CAD build for the part. Positions are in the model's coordinates, mm. Face numbers are marked on the shaded views. Give positions to 0.01 mm unless a question says otherwise; leave off trailing zeros. Loops run counter-clockwise (first coordinate to the right, second up) from the corner with the lowest first, then second, coordinate; pieces in that order, holes last.
```python
from build123d import *

# Parameters (mm, degrees)
SKETCH1_R           = 1
BOSS_EXTRUDE1_DEPTH = 2
SKETCH4_W           = 2
SKETCH4_H           = 2
BOSS_EXTRUDE2_DEPTH = 12


with BuildPart() as part:
    # Sketch1 → Boss-Extrude1 (new body)
    with BuildSketch(Plane(origin=(0, 0, 0), x_dir=(1, 0, 0), z_dir=(0, 1, 0))):
        with BuildLine():
            Line((-10, 2.5), (0, 2.5))
            Line((0, 2.5), (0, -2.5))
            Line((0, -2.5), (-10, -2.5))
            ThreePointArc((-10, -2.5), (-12.5, 0), (-10, 2.5))
        make_face()
        with Locations(Location((-10, 0, 0), (0, 0, 270))):
            Circle(SKETCH1_R, mode=Mode.SUBTRACT)
    extrude(amount=BOSS_EXTRUDE1_DEPTH)

    # Sketch4 → Boss-Extrude2 (add)
    with BuildSketch(Plane(origin=(0, 0, 0), x_dir=(0, 0, -1), z_dir=(1, 0, 0))):
        with Locations((0, 1)):
            Rectangle(SKETCH4_W, SKETCH4_H)
    extrude(amount=BOSS_EXTRUDE2_DEPTH)

    # Sketch5 → Revolve1 (revolve)
    with BuildSketch(Plane.XY):
        with BuildLine():
            Line((10.614180701, 1.574025149), (12, 1))
            Line((12, 1), (13.5, 1))
            ThreePointArc((13.5, 1), (12.292635483, 2.471177921), (10.614180701, 1.574025149))
        make_face()
    revolve(axis=Axis((0.012505213, 1, 0), (1, 0, 0)))


solid = part.part
```
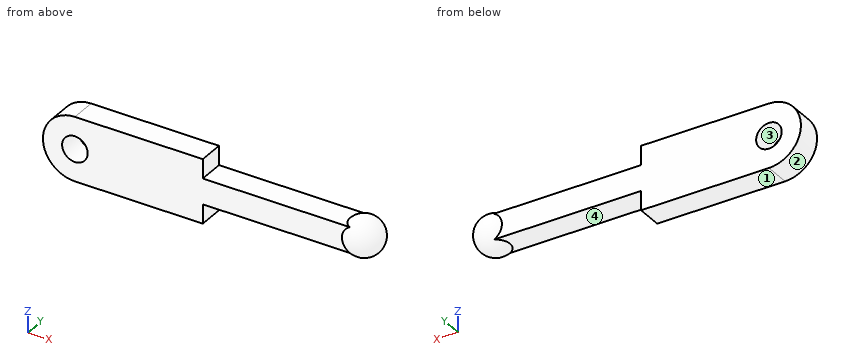
1. Drop flat-ended pins along their axis: pin 1 (1.5 mm diameter, centred on x = 4, z = 0.5, fed in from +Y); pin 2 (1.6 mm diameter, centred on y = 1, z = 2, fed in from +X); pin 3 (1 mm diameter, centred on x = 7.5, y = 1.5, fed in from -Z). Give the stop position or say it passes through.
Responses:
pin 1: stops at y = 2
pin 2: stops at x = 12.9
pin 3: stops at z = -1
2. Probe line 1 along Z through (x, y) = (11, 0.1); line 2 along Y through (x, z) = (-0.5, 1.9); line 3 along X through (y, z) = (1.25, 0.85). List the from-to ranges inside material, lowest first.
Responses:
line 1: z = -1 to 1
line 2: y = 0 to 2
line 3: x = -12.35 to -10.53, -9.47 to 13.21
3. Pull direction X, two halves, no side cores. Call the marked faces 1, 2, 3 and 4: released by +X, released by -X, zero draft, split by the parting line, or undercut.
Responses:
face 1: zero draft
face 2: released by -X
face 3: undercut
face 4: undercut
4. Saw through at A-A, the plane z = 0. List the corners of the cut face in (x, y).
Responses:
outline: (-12.5, 0) - (-11, 0) - (-11, 2) - (-12.5, 2) - close; (-9, 0) - (10.88, 0) arc R1.5 ccw (long way) to (10.88, 2) - (-9, 2) - close
5. Saw through at D-D, the plane y = -0.25. List the corners of the cut face in (x, z).
Responses:
outline: circle Ø1.66 at (12, 0)
6. Saw through at C-C, the plane x = 7.5. List the corners of the cut face in (y, z), and give its area (3 significant figures).
Responses:
outline: (0, -1) - (2, -1) - (2, 1) - (0, 1) - close
area: 4.00 mm2
7. Saw through at B-B, the plane y = 1.45. List the corners of the cut face in (x, z).
Responses:
outline: (-10, -2.5) - (0, -2.5) - (0, -1) - (10.98, -1) arc R1.43 ccw (long way) to (10.98, 1) - (0, 1) - (0, 2.5) - (-10, 2.5) arc R2.5 ccw to start; hole circle Ø2 at (-10, 0)
